Can you work these out from the model? Positions are in its coordinate system, mm. Round coordinates to 2 decimals unless told otherwise and drop trailing zeros. Write each loop counter-clockwise with the first axis right and the second up, starting at its lowest first coordinate (ties: lowest second). Pieces come first, ordered by that corner, then holes. Notation, with made-up numbers: (-0.5, -36.75) - (10.5, -36.75) arc R25 ccw to (10.5, -3.75) - close; hole circle Ø4 at (83, 39). An arc over 180 degrees is marked (long way). One line per item, written item: value. Start each with the question number.
(1) I want a section at A-A on z = 1. List the corners of the cut face in (x, y) for me, plus the area to 3 significant figures.
(2) If I drill on L1, parallel to Y at x = 75, z = 1.1; L2, parallel to X at y = 15, z = 0.2, over which ranges is the centre line in solid material (lowest first)? Write a range as from..to.
(3) I want a section at C-C on x = 117. List the corners of the cut face in (y, z) for me.
(4) I want a section at B-B on y = 36. List the corners of the cut face in (x, z) for me, plus the area to 3 significant figures.
(5) I'm going to push a flat-ended pin straight in: pin 1 Ø1 at (y, z) = (11.5, 1.5) entering from -X. Where does the tip first touch, or does it pass through?
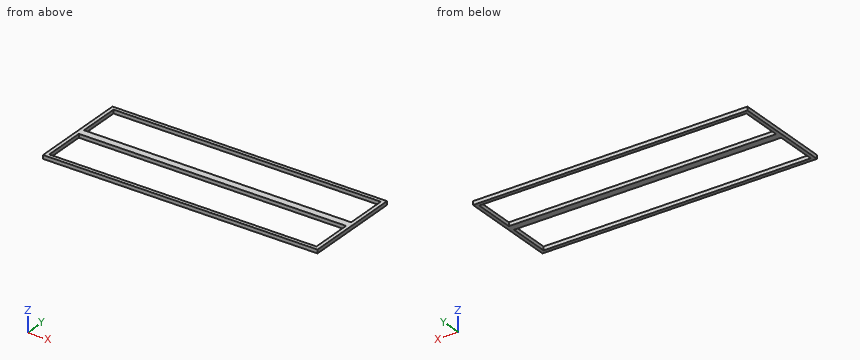
Autodesk Inventor part; units mm, degrees
ref_plane "YZ Plane" through (0, 0, 0) normal (1, 0, 0) x (0, 1, 0)
ref_plane "XZ Plane" through (0, 0, 0) normal (0, 1, 0) x (-1, 0, 0)
ref_plane "XY Plane" through (0, 0, 0) normal (0, 0, 1) x (1, 0, 0)
sketch "Esboço1" plane through (0, 0, 0) normal (0, 0, 1) x (1, 0, 0)
  line L0 (0, 0) -> (150, 0)
  line L1 (150, 0) -> (150, 27)
  line L2 (150, 27) -> (0, 27)
  line L3 (0, 27) -> (0, 0)
  line L4 (2, 25) -> (148, 25)
  line L5 (148, 25) -> (148, 2)
  line L6 (148, 2) -> (2, 2)
  line L7 (2, 2) -> (2, 25)
  line L8 (0, 27) -> (150, 27) construction
  line L9 (0, 54) -> (150, 54)
  line L10 (150, 54) -> (150, 27)
  line L11 (0, 27) -> (0, 54)
  line L12 (2, 29) -> (148, 29)
  line L13 (148, 29) -> (148, 52)
  line L14 (148, 52) -> (2, 52)
  line L15 (2, 52) -> (2, 29)
  dimension "d6" = 150
  dimension "d7" = 27
  dimension "d8" = 2
  dimension "d9" = 2
  dimension "d10" = 2
  dimension "d11" = 2
extrude "Extrusão1" add sketch "Esboço1" along normal blind 2
properties part number "Grade"
Established:
1. outline: (0, 0) - (150, 0) - (150, 54) - (0, 54) - close; hole (2, 2) - (148, 2) - (148, 25) - (2, 25) - close; hole (2, 29) - (148, 29) - (148, 52) - (2, 52) - close
1. area: 1,380 mm2
2. L1: 0..2, 25..29, 52..54
2. L2: 0..2, 148..150
3. outline: (0, 0) - (2, 0) - (2, 2) - (0, 2) - close; (25, 0) - (29, 0) - (29, 2) - (25, 2) - close; (52, 0) - (54, 0) - (54, 2) - (52, 2) - close
4. outline: (0, 0) - (2, 0) - (2, 2) - (0, 2) - close; (148, 0) - (150, 0) - (150, 2) - (148, 2) - close
4. area: 8.00 mm2
5. pin 1: x = 0
